Part model, mm, in its own coordinate system. Round coordinates to 2 decimals unless told otherwise and drop trailing zeros. Write each loop counter-clockwise with the first axis right and the second up, starting at its lowest first coordinate (ties: lowest second). Pieces come first, ordered by that corner, then holes. Notation, with made-up numbers: M 48.25,-34 L 88.25,-34 A21 ccw 88.25,0 Z; hole C 32,22.25 d4. An arc over 180 degrees is marked long. Use a Markdown table: item, result. Add a question column.
1) Drop flat-ended pins along their axis: P1, Ø12, axis at x = 15, z = -277, coming from the -Y side; P2, Ø12, axis at x = -4.5, z = -147.5, coming from the +Y side. Give the stop position or say it passes through.
2) Wall check: probe 1 along Z at (x, y) = (-0.5, -586); probe 2 along Z at (x, y) = (1.5, -479); probe 3 along Y at (x, z) = (0, -38). Give the ranges that are in metal, low to high.
3) Slice it at A-A on y = 0. Write the cut outline in (x, z).
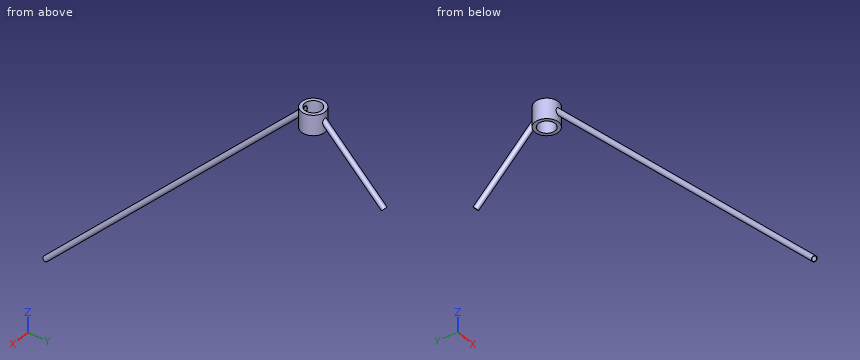
```python
from build123d import *

# Parameters (mm, degrees)
F2_R     = 8
F2_R_2   = 7
F4_R     = 25
F5_DEPTH = 40
F7_START = -5
F6_R     = 35
F6_R_2   = 25
F7_DEPTH = 60


with BuildPart() as f3:
    # F3: sweep along a path in F0
    with BuildLine(Plane.YZ) as f3_path:
        Line((-800, -800), (0, 0))
        Line((0, 0), (212.132034356, -212.132034356))
    # F2 (on line) → F3 (sweep)
    with BuildSketch(Plane(origin=(0, -800, -800), x_dir=(1, 0, 0), z_dir=(0, -0.7071067812, -0.7071067812))):
        Circle(F2_R)
        Circle(F2_R_2, mode=Mode.SUBTRACT)
    sweep(path=f3_path.line, transition=Transition.RIGHT)

    # F4 (on Top) → F5 (cut, symmetric)
    with BuildSketch(Plane.XY):
        Circle(F4_R)
    extrude(amount=F5_DEPTH, both=True, mode=Mode.SUBTRACT)

    # F6 (on Top) → F7 (join)
    with BuildSketch(Plane.XY.offset(F7_START)):
        Circle(F6_R)
        Circle(F6_R_2, mode=Mode.SUBTRACT)
    extrude(amount=-F7_DEPTH)


solid = f3.part
```
Entries:
| question | item | result |
|---|---|---|
| 1 | P1 | passes through |
| 1 | P2 | stops at y = 163.92 |
| 2 | probe 1 | z = -597.29 to -595.87, -576.13 to -574.71 |
| 2 | probe 2 | z = -490.11 to -488.67, -469.33 to -467.89 |
| 2 | probe 3 | y = -49.31 to -47.9, -35 to -25, 25 to 35, 47.9 to 49.31 |
| 3 | outline | M -35,-65 L -25,-65 L -25,-5 L -35,-5 Z; M 25,-65 L 35,-65 L 35,-5 L 25,-5 Z |
